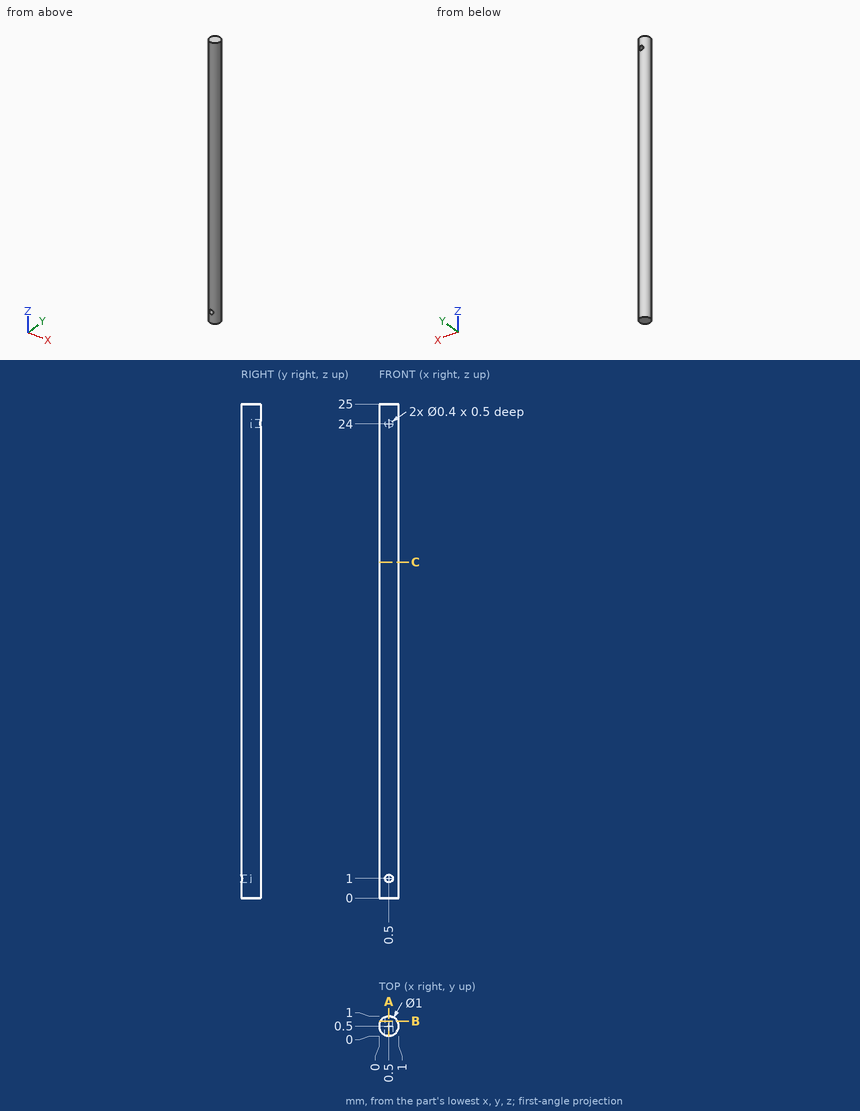
For this review, use the dimensioned drawing (mm, ordinates from the lowest corner) and the shaded views. Give positions to 0.01 mm unless a question says otherwise; leave off trailing zeros. Write each loop counter-clockwise with the first axis right and the second up, starting at its lowest first coordinate (ties: lowest second). Pieces come first, ordered by that corner, then holes.
(1) Consider section C-C, the plane z = 17. Give the boundary of the cut face in (x, y), and give its area (3 significant figures).
(2) Consider section B-B, the plane y = 0.75. Give the boundary of the cut face in (x, z), and give its area (3 significant figures).
(3) Consider section A-A, the plane x = 0.5. Give the boundary of the cut face in (y, z), and give its area (3 significant figures).
(4) To check wall thickness, follow L1, parallel to Z at x = 0.5, y = 0.45; L2, parallel to Z at x = 0.5, y = 0.6; L3, parallel to Y at x = 0.55, z = 18.5. State the ranges of each line that lie inside material, in increasing order.
Returned:
1. outline: circle Ø1 at (0.5, 0.5)
1. area: 0.785 mm2
2. outline: (0.07, 0) - (0.93, 0) - (0.93, 25) - (0.07, 25) - close; hole circle Ø0.4 at (0.5, 24)
2. area: 21.5 mm2
3. outline: (0, 0) - (1, 0) - (1, 23.8) - (0.5, 23.8) - (0.5, 24.2) - (1, 24.2) - (1, 25) - (0, 25) - (0, 1.2) - (0.5, 1.2) - (0.5, 0.8) - (0, 0.8) - close
3. area: 24.6 mm2
4. L1: z = 0 to 0.8, 1.2 to 25
4. L2: z = 0 to 23.8, 24.2 to 25
4. L3: y = 0 to 1
